CAD build for the part. Positions are in the model's coordinates, mm. Face numbers are marked on the shaded views. Coordinates: 2 decimals unless noted, no trailing zeros. Order: outer loops, then holes, each group sorted by start corner. A loop starts at its lowest first (then second) coordinate and runs counter-clockwise, first axis right, second up. Notation, with made-up numbers: (-5.5, 51.25) -> (4.5, 51.25) arc R20 ccw to (4.5, 73.25) -> close; hole circle Ø5 at (22, 82). An arc over 180 degrees is marked (long way). Use one line per item in the form item = value. Start each with the question number.
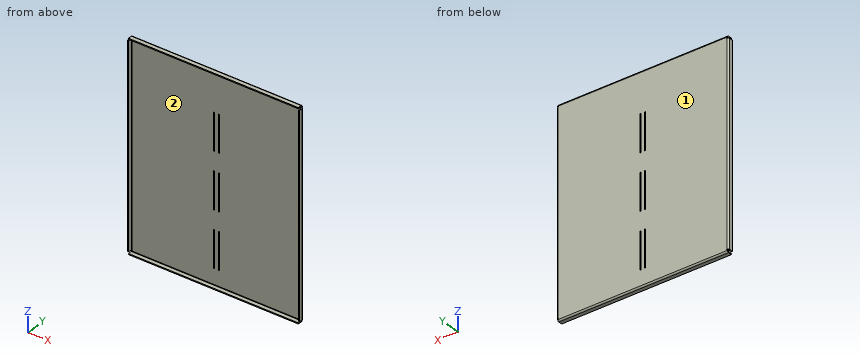
from build123d import *

# Parameters (mm, degrees)
SKETCH1_W                     = 325
SKETCH1_H                     = 10
BASE_FLANGE1_DEPTH            = 2
EDGE_FLANGE1_STRIP_W          = 9.4732
EDGE_FLANGE1_STRIP_H          = 2
EDGE_FLANGE1_STRIP_CUT_DEPTH  = 325
EDGE_FLANGE1_DEPTH            = 325
EDGE_FLANGE2_STRIP_W          = 9.4732
EDGE_FLANGE2_STRIP_H          = 2
EDGE_FLANGE2_STRIP_CUT_DEPTH  = 325
EDGE_FLANGE2_DEPTH            = 325
EDGE_FLANGE3_STRIP_W          = 9.4732
EDGE_FLANGE3_STRIP_H          = 2
EDGE_FLANGE3_STRIP_CUT_DEPTH  = 377.9268
EDGE_FLANGE3_RELIEF_W         = 10.4732
EDGE_FLANGE3_RELIEF_H         = 1
EDGE_FLANGE3_RELIEF_CUT_DEPTH = 2
EDGE_FLANGE3_DEPTH            = 377.9268
EDGE_FLANGE4_STRIP_W          = 9.4732
EDGE_FLANGE4_STRIP_H          = 2
EDGE_FLANGE4_STRIP_CUT_DEPTH  = 377.9268
EDGE_FLANGE4_RELIEF_W         = 10.4732
EDGE_FLANGE4_RELIEF_H         = 1
EDGE_FLANGE4_RELIEF_CUT_DEPTH = 2
EDGE_FLANGE4_DEPTH            = 377.9268
CUT_EXTRUDE1_DEPTH            = 421.997636573
CUT_EXTRUDE1_DEPTH_BACK       = 421.997636573
SKETCH14_W                    = 2
SKETCH14_H                    = 70


# Sheet-metal steps are written as plain solids
with BuildPart() as part:
    # Sketch1 → Base-Flange1 (new body)
    with BuildSketch(Plane.XY):
        Rectangle(SKETCH1_W, SKETCH1_H)
    extrude(amount=-BASE_FLANGE1_DEPTH)

    # Edge-Flange1 strip (across the edge) → Edge-Flange1 strip cut (cut)
    with BuildSketch(Plane(origin=(-162.5, 5, -2), x_dir=(0, -1, 0), z_dir=(1, 0, 0))):
        with Locations((-2, -1)):
            Rectangle(EDGE_FLANGE1_STRIP_W, EDGE_FLANGE1_STRIP_H)
    extrude(amount=EDGE_FLANGE1_STRIP_CUT_DEPTH, mode=Mode.SUBTRACT)

    # Edge-Flange1 section (across the edge) → Edge-Flange1 (add)
    with BuildSketch(Plane(origin=(-162.5, 5, -2), x_dir=(0, -1, 0), z_dir=(1, 0, 0))):
        with BuildLine():
            Line((0, 0.7366), (0, 385.4))
            Line((0, 385.4), (2, 385.4))
            Line((2, 385.4), (2, 0.7366))
            ThreePointArc((2, 0.7366), (2.215745145, 0.215745145), (2.7366, 0))
            Line((2.7366, 0), (2.7366, -2))
            ThreePointArc((2.7366, -2), (0.801531583, -1.198468417), (0, 0.7366))
        make_face()
    extrude(amount=EDGE_FLANGE1_DEPTH)

    # Edge-Flange2 strip (across the edge) → Edge-Flange2 strip cut (cut)
    with BuildSketch(Plane(origin=(-162.5, 3, -387.4), x_dir=(0, 0, 1), z_dir=(1, 0, 0))):
        with Locations((-2, -1)):
            Rectangle(EDGE_FLANGE2_STRIP_W, EDGE_FLANGE2_STRIP_H)
    extrude(amount=EDGE_FLANGE2_STRIP_CUT_DEPTH, mode=Mode.SUBTRACT)

    # Edge-Flange2 section (across the edge) → Edge-Flange2 (add)
    with BuildSketch(Plane(origin=(-162.5, 3, -387.4), x_dir=(0, 0, 1), z_dir=(1, 0, 0))):
        with BuildLine():
            Line((0, 0.7366), (0, 8))
            Line((0, 8), (2, 8))
            Line((2, 8), (2, 0.7366))
            ThreePointArc((2, 0.7366), (2.215745145, 0.215745145), (2.7366, 0))
            Line((2.7366, 0), (2.7366, -2))
            ThreePointArc((2.7366, -2), (0.801531583, -1.198468417), (0, 0.7366))
        make_face()
    extrude(amount=EDGE_FLANGE2_DEPTH)

    # Edge-Flange3 strip (across the edge) → Edge-Flange3 strip cut (cut)
    with BuildSketch(Plane(origin=(162.5, 3, -382.6634), x_dir=(-1, 0, 0), z_dir=(0, 0, 1))):
        with Locations((-4, -1)):
            Rectangle(EDGE_FLANGE3_STRIP_W, EDGE_FLANGE3_STRIP_H)
    extrude(amount=EDGE_FLANGE3_STRIP_CUT_DEPTH, mode=Mode.SUBTRACT)

    # Edge-Flange3 relief (on the sheet) → Edge-Flange3 relief cut (cut)
    with BuildSketch(Plane(origin=(161.7634, 3, -382.6634), x_dir=(-1, 0, 0), z_dir=(0, -1, 0))):
        with Locations((-4.2366, 0.5)):
            Rectangle(EDGE_FLANGE3_RELIEF_W, EDGE_FLANGE3_RELIEF_H)
        with Locations((-4.2366, -378.4268)):
            Rectangle(EDGE_FLANGE3_RELIEF_W, EDGE_FLANGE3_RELIEF_H)
    extrude(amount=-EDGE_FLANGE3_RELIEF_CUT_DEPTH, mode=Mode.SUBTRACT)

    # Edge-Flange3 section (across the edge) → Edge-Flange3 (add)
    with BuildSketch(Plane(origin=(162.5, 3, -382.6634), x_dir=(-1, 0, 0), z_dir=(0, 0, 1))):
        with BuildLine():
            Line((-2, 0.7366), (-2, 8))
            Line((-2, 8), (0, 8))
            Line((0, 8), (0, 0.7366))
            ThreePointArc((0, 0.7366), (0.215745145, 0.215745145), (0.7366, 0))
            Line((0.7366, 0), (0.7366, -2))
            ThreePointArc((0.7366, -2), (-1.198468417, -1.198468417), (-2, 0.7366))
        make_face()
    extrude(amount=EDGE_FLANGE3_DEPTH)

    # Edge-Flange4 strip (across the edge) → Edge-Flange4 strip cut (cut)
    with BuildSketch(Plane(origin=(-162.5, 3, -4.7366), x_dir=(1, 0, 0), z_dir=(0, 0, -1))):
        with Locations((-4, -1)):
            Rectangle(EDGE_FLANGE4_STRIP_W, EDGE_FLANGE4_STRIP_H)
    extrude(amount=EDGE_FLANGE4_STRIP_CUT_DEPTH, mode=Mode.SUBTRACT)

    # Edge-Flange4 relief (on the sheet) → Edge-Flange4 relief cut (cut)
    with BuildSketch(Plane(origin=(-161.7634, 3, -4.7366), x_dir=(1, 0, 0), z_dir=(0, -1, 0))):
        with Locations((-4.2366, 0.5)):
            Rectangle(EDGE_FLANGE4_RELIEF_W, EDGE_FLANGE4_RELIEF_H)
        with Locations((-4.2366, -378.4268)):
            Rectangle(EDGE_FLANGE4_RELIEF_W, EDGE_FLANGE4_RELIEF_H)
    extrude(amount=-EDGE_FLANGE4_RELIEF_CUT_DEPTH, mode=Mode.SUBTRACT)

    # Edge-Flange4 section (across the edge) → Edge-Flange4 (add)
    with BuildSketch(Plane(origin=(-162.5, 3, -4.7366), x_dir=(1, 0, 0), z_dir=(0, 0, -1))):
        with BuildLine():
            Line((-2, 0.7366), (-2, 8))
            Line((-2, 8), (0, 8))
            Line((0, 8), (0, 0.7366))
            ThreePointArc((0, 0.7366), (0.215745145, 0.215745145), (0.7366, 0))
            Line((0.7366, 0), (0.7366, -2))
            ThreePointArc((0.7366, -2), (-1.198468417, -1.198468417), (-2, 0.7366))
        make_face()
    extrude(amount=EDGE_FLANGE4_DEPTH)

    # Sketch14 → Cut-Extrude1 (cut, two sides: drawn at the far end of the back side and taken through both)
    with BuildSketch(Plane(origin=(0, 5, 0), x_dir=(1, 0, 0), z_dir=(0, 1, 0)).offset(-CUT_EXTRUDE1_DEPTH_BACK)):
        with Locations((-4.5, 321.2)):
            Rectangle(SKETCH14_W, SKETCH14_H)
        with Locations((4.5, 321.2)):
            Rectangle(SKETCH14_W, SKETCH14_H)
        with Locations((-4.5, 216.2)):
            Rectangle(SKETCH14_W, SKETCH14_H)
        with Locations((4.5, 216.2)):
            Rectangle(SKETCH14_W, SKETCH14_H)
        with Locations((-4.5, 111.2)):
            Rectangle(SKETCH14_W, SKETCH14_H)
        with Locations((4.5, 111.2)):
            Rectangle(SKETCH14_W, SKETCH14_H)
    extrude(amount=CUT_EXTRUDE1_DEPTH + CUT_EXTRUDE1_DEPTH_BACK, mode=Mode.SUBTRACT)


solid = part.part
1) Drop flat-ended pins along their axis: P1, Ø1.6, axis at x = -4.5, y = 4, coming from the +Z side; P2, Ø5, axis at x = -30.5, z = -266.5, coming from the -Y side; P3, Ø2, axis at y = 4, z = -112, coming from the +X side. Give the stop position or say it passes through.
2) Cut at B-B on z = -323.5. Give the cut face in (x, y), then the cut area to 3 significant figures.
3) Cut at D-D on z = -172. Give the cut face in (x, y), then the cut area to 3 significant figures.
4) Cut at C-C on x = -27. Give the cut face in (y, z).
5) Two-plate mould, pull along Z, no slides. Class the marked faces 1 and 2: released by +Z, released by -Z, zero draft, split by the parting line, or undercut.
6) Cut at A-A on y = 0.25. Give the cut face in (x, z), then the cut area to 3 significant figures.
7) Probe L1, parallel to X at y = -1, z = -214; L2, parallel to Z at x = 61, y = -3.5; L3, parallel to Y at x = -117, z = -112.5. List the from-to ranges inside material, lowest first.
Values follow:
q1.P1 = -0.17
q1.P2 = 3
q1.P3 = 164.4
q2.outline = (-164.5, -5) -> (-162.5, -5) -> (-162.5, 2.26) arc R0.74 cw to (-161.76, 3) -> (-5.5, 3) -> (-5.5, 5) -> (-161.76, 5) arc R2.74 ccw to (-164.5, 2.26) -> close; (-3.5, 3) -> (3.5, 3) -> (3.5, 5) -> (-3.5, 5) -> close; (5.5, 3) -> (161.76, 3) arc R0.74 cw to (162.5, 2.26) -> (162.5, -5) -> (164.5, -5) -> (164.5, 2.26) arc R2.74 ccw to (161.76, 5) -> (5.5, 5) -> close
q2.area = 679 mm^2
q3.outline = (-164.5, -5) -> (-162.5, -5) -> (-162.5, 2.26) arc R0.74 cw to (-161.76, 3) -> (161.76, 3) arc R0.74 cw to (162.5, 2.26) -> (162.5, -5) -> (164.5, -5) -> (164.5, 2.26) arc R2.74 ccw to (161.76, 5) -> (-161.76, 5) arc R2.74 ccw to (-164.5, 2.26) -> close
q3.area = 687 mm^2
q4.outline = (-5, -387.4) -> (2.26, -387.4) arc R2.74 ccw to (5, -384.66) -> (5, -2.74) arc R2.74 ccw to (2.26, 0) -> (-5, 0) -> (-5, -2) -> (2.26, -2) arc R0.74 cw to (3, -2.74) -> (3, -384.66) arc R0.74 cw to (2.26, -385.4) -> (-5, -385.4) -> close
q5.face_1 = zero draft
q5.face_2 = undercut
q6.outline = (-164.5, -382.66) -> (-162.5, -382.66) -> (-162.5, -4.74) -> (-164.5, -4.74) -> close; (-162.5, -387.4) -> (162.5, -387.4) -> (162.5, -385.4) -> (-162.5, -385.4) -> close; (-162.5, -2) -> (162.5, -2) -> (162.5, 0) -> (-162.5, 0) -> close; (162.5, -382.66) -> (164.5, -382.66) -> (164.5, -4.74) -> (162.5, -4.74) -> close
q6.area = 2,810 mm^2
q7.L1 = -164.5 to -162.5, 162.5 to 164.5
q7.L2 = -387.4 to -385.4, -2 to 0
q7.L3 = 3 to 5
